Verification items for the finished model (mm, model axes). Face numbers are marked on the shaded views. A direction names the side the tool comes from. Give positions to 0.01 mm unless a question says otherwise; leave off trailing zeros. Order: outer loops, then holes, each group sorted by start corner. A loop starts at its lowest first (then second) coordinate and runs counter-clockwise, first axis right, second up. Notation, with made-up numbers: (84.25, 14.5) -> (138.25, 14.5) arc R18 cw to (138.25, 28.5) -> close; hole circle Ø9 at (36, -11). An arc over 180 degrees is marked (long way). Return JSON: item names as keys, results as strings. Group by question number.
(1) Cross-section at A-A on z = 24. Enter the section's corners in (x, y), then the cut area to 3 significant figures.
(2) Tool access check on the marked faces 1, 2, 3 and 4. Record the directions out of +Z, -Z, +X, -X, +Y, -Y that give a thin tool (end or side, any length) a straight path to the whole face; none if there is none.
(3) Cross-section at C-C on y = 43. Enter the section's corners in (x, z).
(4) Release check for a two-part mould opening along X. For the marked faces 5, 6 and 7 record: pulls with the +X half, pulls with the -X half, needs draft (parallel to the pull), parting line crosses it, or undercut.
(5) Cross-section at D-D on y = 14. Enter the section's corners in (x, z).
(6) Cross-section at B-B on x = 15. Enter the section's corners in (y, z).
(7) Thickness scan on line 1 along X through (y, z) = (8.5, -8.5); line 2 along Z through (x, y) = (-62, 22); line 3 along Z through (x, y) = (-41, 19.5). Record the ranges inside material, lowest first.
(8) Depth check by flat-ended pin: pin 1 Ø5 at (y, z) = (15, -37.5) entering from -X; pin 2 Ø1.5 at (x, z) = (47.5, 28) entering from +Y; pin 3 Ø1.5 at (x, y) = (34, 2) entering from -Z. Enter the tip coordinate at first touch or a pass-through.
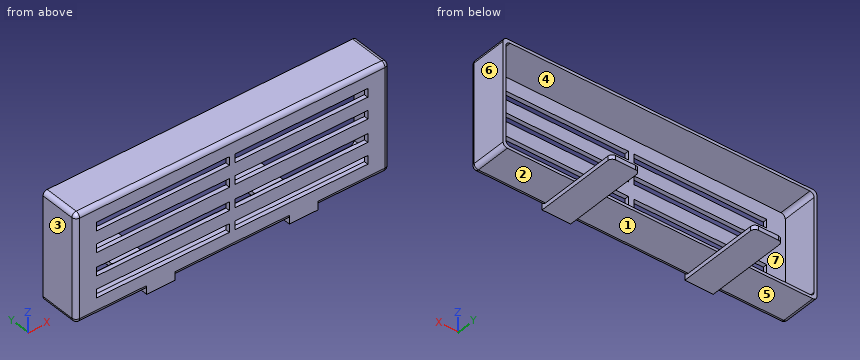
from build123d import *

# Parameters (mm, degrees)
SKIZZE1_W                       = 220
SKIZZE1_H                       = 75
AUFSATZ_LINEAR_AUSTRAGEN1_DEPTH = 3
SKIZZE3_W                       = 20
SKIZZE3_H                       = 3
AUFSATZ_LINEAR_AUSTRAGEN3_DEPTH = 60
SKIZZE4_W                       = 220
SKIZZE4_H                       = 75
AUFSATZ_LINEAR_AUSTRAGEN4_DEPTH = 25
SKIZZE5_W                       = 190
SKIZZE5_H                       = 6
SCHNITT_LINEAR_AUSTRAGEN1_DEPTH = 131.342817217
SKIZZE6_W                       = 4
SKIZZE6_H                       = 52
AUFSATZ_LINEAR_AUSTRAGEN5_DEPTH = 3
VERRUNDUNG1_R                   = 3
VERRUNDUNG2_R                   = 3
VERRUNDUNG3_R                   = 3
VERRUNDUNG4_R                   = 3


with BuildPart() as part:
    # Skizze1 → Aufsatz-Linear austragen1 (new body)
    with BuildSketch(Plane(origin=(0, 0, 0), x_dir=(1, 0, 0), z_dir=(0, 1, 0))):
        Rectangle(SKIZZE1_W, SKIZZE1_H)
    extrude(amount=AUFSATZ_LINEAR_AUSTRAGEN1_DEPTH)

    # Skizze3 → Aufsatz-Linear austragen3 (add)
    with BuildSketch(Plane(origin=(0, 0, 0), x_dir=(1, 0, 0), z_dir=(0, 1, 0))):
        with Locations((50, 39)):
            Rectangle(SKIZZE3_W, SKIZZE3_H)
        with Locations((-50, 39)):
            Rectangle(SKIZZE3_W, SKIZZE3_H)
    extrude(amount=AUFSATZ_LINEAR_AUSTRAGEN3_DEPTH)

    # Skizze4 → Aufsatz-Linear austragen4 (add)
    with BuildSketch(Plane(origin=(0, 3, 0), x_dir=(1, 0, 0), z_dir=(0, 1, 0))):
        Rectangle(SKIZZE4_W, SKIZZE4_H)
        Polygon((108, 35.5), (60, 35.5), (40, 35.5), (-40, 35.5), (-60, 35.5), (-108, 35.5), (-108, -35.5), (108, -35.5), align=None, mode=Mode.SUBTRACT)
    extrude(amount=AUFSATZ_LINEAR_AUSTRAGEN4_DEPTH)

    # Skizze5 → Schnitt-Linear austragen1 (cut, through all)
    with BuildSketch(Plane(origin=(0, 3, 0), x_dir=(1, 0, 0), z_dir=(0, 1, 0))):
        with Locations((0, 23)):
            Rectangle(SKIZZE5_W, SKIZZE5_H)
        with Locations((0, 8)):
            Rectangle(SKIZZE5_W, SKIZZE5_H)
        with Locations((0, -8)):
            Rectangle(SKIZZE5_W, SKIZZE5_H)
        with Locations((0, -23)):
            Rectangle(SKIZZE5_W, SKIZZE5_H)
    extrude(amount=-SCHNITT_LINEAR_AUSTRAGEN1_DEPTH, mode=Mode.SUBTRACT)

    # Skizze6 → Aufsatz-Linear austragen5 (add, through all)
    with BuildSketch(Plane(origin=(0, 3, 0), x_dir=(1, 0, 0), z_dir=(0, 1, 0))):
        Rectangle(SKIZZE6_W, SKIZZE6_H)
    extrude(amount=-AUFSATZ_LINEAR_AUSTRAGEN5_DEPTH)

    # Verrundung1
    verrundung1_edges = [part.edges().sort_by_distance(p)[0] for p in [
        (40, 60, -39),
        (60, 60, -39),
        (-40, 60, -39),
        (-60, 60, -39),
    ]]
    fillet(verrundung1_edges, radius=VERRUNDUNG1_R)

    # Verrundung2
    verrundung2_edges = [part.edges().sort_by_distance(p)[0] for p in [
        (108, 15.5, -35.5),
        (-108, 15.5, -35.5),
        (-108, 15.5, 35.5),
        (108, 15.5, 35.5),
        (110, 14, -37.5),
        (110, 14, 37.5),
        (-110, 14, 37.5),
        (-110, 14, -37.5),
    ]]
    fillet(verrundung2_edges, radius=VERRUNDUNG2_R)

    # Verrundung3
    verrundung3_edges = [part.edges().sort_by_distance(p)[0] for p in [
        (-110, 0, 0),
        (83.5, 0, -37.5),
        (110, 0, 0),
        (0, 0, 37.5),
        (109.121320344, 0, 36.621320344),
        (109.121320344, 0, -36.621320344),
        (-109.121320344, 0, 36.621320344),
        (-109.121320344, 0, -36.621320344),
        (-83.5, 0, -37.5),
    ]]
    fillet(verrundung3_edges, radius=VERRUNDUNG3_R)

    # Verrundung4
    verrundung4_edges = [part.edges().sort_by_distance(p)[0] for p in [
        (0, 0, -37.5),
    ]]
    fillet(verrundung4_edges, radius=VERRUNDUNG4_R)


solid = part.part
Verdict:
{
 "1": {"outline": "(-110, 3) arc R3 ccw to (-107, 0) -> (-95, 0) -> (-95, 3) -> (-108, 3) -> (-108, 28) -> (-110, 28) -> close; (-2, 0) -> (2, 0) -> (2, 3) -> (-2, 3) -> close; (95, 0) -> (107, 0) arc R3 ccw to (110, 3) -> (110, 28) -> (108, 28) -> (108, 3) -> (95, 3) -> close", "area": "198 mm²"},
 "2": {"face 1": "-Z, +Y, -Y", "face 2": "-Z, +X, +Y, -Y", "face 3": "+Z, -Z, -X, +Y, -Y", "face 4": "+Y"},
 "3": {"outline": "(-60, -40.5) -> (-40, -40.5) -> (-40, -37.5) -> (-60, -37.5) -> close; (40, -40.5) -> (60, -40.5) -> (60, -37.5) -> (40, -37.5) -> close"},
 "4": {"face 5": "needs draft", "face 6": "pulls with the +X half", "face 7": "undercut"},
 "5": {"outline": "(-110, -34.5) arc R3 ccw to (-107, -37.5) -> (-60, -37.5) -> (-60, -40.5) -> (-40, -40.5) -> (-40, -37.5) -> (40, -37.5) -> (40, -40.5) -> (60, -40.5) -> (60, -37.5) -> (107, -37.5) arc R3 ccw to (110, -34.5) -> (110, 34.5) arc R3 ccw to (107, 37.5) -> (-107, 37.5) arc R3 ccw to (-110, 34.5) -> close; hole (-108, -32.5) arc R3 ccw to (-105, -35.5) -> (105, -35.5) arc R3 ccw to (108, -32.5) -> (108, 32.5) arc R3 ccw to (105, 35.5) -> (-105, 35.5) arc R3 ccw to (-108, 32.5) -> close"},
 "6": {"outline": "(0, -34.5) arc R3 ccw to (3, -37.5) -> (28, -37.5) -> (28, -35.5) -> (3, -35.5) -> (3, -26) -> (0, -26) -> close; (0, -20) -> (3, -20) -> (3, -11) -> (0, -11) -> close; (0, -5) -> (3, -5) -> (3, 5) -> (0, 5) -> close; (0, 11) -> (3, 11) -> (3, 20) -> (0, 20) -> close; (0, 26) -> (3, 26) -> (3, 35.5) -> (28, 35.5) -> (28, 37.5) -> (3, 37.5) arc R3 ccw to (0, 34.5) -> close"},
 "7": {"line 1": "-110 to -108, 108 to 110", "line 2": "-37.5 to -35.5, 35.5 to 37.5", "line 3": "-40.5 to -35.5, 35.5 to 37.5"},
 "8": {"pin 1": "x = -109.96", "pin 2": "y = 3", "pin 3": "z = -37.49"}
}
